from build123d import *

# Parameters (mm, degrees)
SKETCH1_W           = 40
SKETCH1_H           = 60
BOSS_EXTRUDE1_DEPTH = 3.05
SKETCH4_W           = 3.3
SKETCH4_H           = 52
SKETCH4_W_2         = 3
SKETCH4_H_2         = 0.8
CUT_EXTRUDE1_DEPTH  = 10
SKETCH7_R           = 8
CUT_EXTRUDE4_DEPTH  = 10
SKETCH8_R           = 1.5
CUT_EXTRUDE5_DEPTH  = 10
FILLET1_R           = 0.5


with BuildPart() as part:
    # Sketch1 → Boss-Extrude1 (new body)
    with BuildSketch(Plane(origin=(0, 0, 0), x_dir=(1, 0, 0), z_dir=(0, 1, 0))):
        with Locations((20, 30)):
            Rectangle(SKETCH1_W, SKETCH1_H)
    extrude(amount=BOSS_EXTRUDE1_DEPTH)

    # Sketch4 → Cut-Extrude1 (cut)
    with BuildSketch(Plane(origin=(0, 3.05, 0), x_dir=(1, 0, 0), z_dir=(0, 1, 0))):
        with Locations((20, 30)):
            Rectangle(SKETCH4_W, SKETCH4_H)
        with Locations((20, 57.6)):
            Rectangle(SKETCH4_W_2, SKETCH4_H_2)
    extrude(amount=-CUT_EXTRUDE1_DEPTH, mode=Mode.SUBTRACT)

    # Sketch7 → Cut-Extrude4 (cut)
    with BuildSketch(Plane(origin=(0, 3.05, 0), x_dir=(1, 0, 0), z_dir=(0, 1, 0))):
        with Locations((8, 35)):
            Circle(SKETCH7_R)
        with Locations((8, 49)):
            Circle(SKETCH7_R)
        with BuildLine():
            Line((8, 57), (0, 57))
            Line((0, 57), (0, 49))
            ThreePointArc((0, 49), (2.343145751, 54.656854249), (8, 57))
        make_face()
        with BuildLine():
            Line((16, 35), (16, 49))
            ThreePointArc((16, 49), (14.891439137, 44.936987987), (11.872983346, 42))
            ThreePointArc((11.872983346, 42), (14.891439137, 39.063012013), (16, 35))
        make_face()
        with BuildLine():
            ThreePointArc((4.127016654, 42), (1.108560863, 44.936987987), (0, 49))
            Line((0, 49), (0, 35))
            ThreePointArc((0, 35), (1.108560863, 39.063012013), (4.127016654, 42))
        make_face()
        with BuildLine():
            ThreePointArc((8, 27), (2.343145751, 29.343145751), (0, 35))
            Line((0, 35), (0, 27))
            Line((0, 27), (8, 27))
        make_face()
        with BuildLine():
            ThreePointArc((28.127016654, 42), (25.108560863, 44.936987987), (24, 49))
            Line((24, 49), (24, 35))
            ThreePointArc((24, 35), (25.108560863, 39.063012013), (28.127016654, 42))
        make_face()
        with Locations((32, 35)):
            Circle(SKETCH7_R)
        with Locations((32, 49)):
            Circle(SKETCH7_R)
        with BuildLine():
            Line((40, 35), (40, 49))
            ThreePointArc((40, 49), (38.891439137, 44.936987987), (35.872983346, 42))
            ThreePointArc((35.872983346, 42), (38.891439137, 39.063012013), (40, 35))
        make_face()
        with BuildLine():
            Line((40, 27), (40, 35))
            ThreePointArc((40, 35), (37.656854263, 29.343145764), (32.000000039, 27))
            Line((32.000000039, 27), (40, 27))
        make_face()
        with BuildLine():
            Line((40, 49), (40, 57))
            Line((40, 57), (32, 57))
            ThreePointArc((32, 57), (37.656854249, 54.656854249), (40, 49))
        make_face()
    extrude(amount=-CUT_EXTRUDE4_DEPTH, mode=Mode.SUBTRACT)

    # Sketch8 → Cut-Extrude5 (cut)
    with BuildSketch(Plane(origin=(0, 3.05, 0), x_dir=(1, 0, 0), z_dir=(0, 1, 0))):
        with BuildLine():
            ThreePointArc((9.5, 2.5), (6.939339828, 3.560660172), (8, 1))
            Line((8, 1), (8, 2.5))
            Line((8, 2.5), (9.5, 2.5))
        make_face()
        with BuildLine():
            Line((8, 2.5), (8, 1))
            ThreePointArc((8, 1), (9.060660172, 1.439339828), (9.5, 2.5))
            Line((9.5, 2.5), (8, 2.5))
        make_face()
        with Locations(Location((32, 2.5, 0), (0, 0, 270))):
            Circle(SKETCH8_R)
    extrude(amount=-CUT_EXTRUDE5_DEPTH, mode=Mode.SUBTRACT)

    # Fillet1
    fillet1_edges = [part.edges().sort_by_distance(p)[0] for p in [
        (0, 1.525, -27),
        (0, 1.525, -57),
        (40, 1.525, -57),
        (40, 1.525, -27),
        (0, 1.525, -60),
        (40, 1.525, -60),
    ]]
    fillet(fillet1_edges, radius=FILLET1_R)


solid = part.part
Verification items for the finished model (mm, model axes). A direction names the side the tool comes from. Give positions to 0.01 mm unless a question says otherwise; leave off trailing zeros. Write each loop counter-clockwise with the first axis right and the second up, starting at its lowest first coordinate (ties: lowest second). Pieces come first, ordered by that corner, then holes. Notation, with made-up numbers: M -28,-13 L -13,-13 A14 cw -13,8 Z; hole C 22,43.25 d7. An arc over 180 degrees is marked long. Put each result on its own line as item: value. Start each with the question number.
1. Scan lines: line 1 along Z through (x, y) = (20, 2); line 2 along X through (y, z) = (0.6, -2.5); line 3 along Z through (x, y) = (8, 1.4). Record each from-to range of solid material in increasing order. Write a range as [from, to].
2. Section check B-B (y = 2.25). Give the number of separate pieces and of enclosed holes in the cut face, and give its area (3 significant figures).
3. Section check C-C (z = -12.5). Record the cut outline in (x, y).
4. Draft check along Z on faces 1 (the face through (4, 2, -27)), 2 (the face through (20, 2, -60)), 3 (the face through (0, 2, -58)). Enter one of: +Z half, -Z half, draft (parallel to the pull), parting line (faces both ways), or undercut.
5. Go/stop test with flat-tipped pins: pin 1 Ø0.9 at (y, z) = (1.5, -45) entering from -X; pin 2 Ø1.5 at (y, z) = (2, -31) entering from +X; pin 3 Ø1.5 at (y, z) = (2.5, -39.5) entering from +X. Record where each tip stops, or that it passes through.
6. Set-up check for faces 4 (the face through (36, 2, -27)), 5 (the face through (0, 2, -13)), 6 (the face through (16, 2, -42)), 7 (the face through (20, 2, -58)): record each of +Z, -Z, +X, -X, +Y, -Y from which the full face is reachable in a straight line by a thin tool's end or side.
7. Section check A-A (z = -41). Record the cut outline in (x, y).
Answer list:
1. line 1: [-60, -58], [-57.2, -56], [-4, 0]
1. line 2: [0, 6.5], [9.5, 30.5], [33.5, 40]
1. line 3: [-60, -57], [-27, -4], [-1, 0]
2. separate pieces: 1
2. enclosed holes: 4
2. area: 1,310 mm2
3. outline: M 0,0 L 18.35,0 L 18.35,3.05 L 0,3.05 Z; M 21.65,0 L 40,0 L 40,3.05 L 21.65,3.05 Z
4. face 1: undercut
4. face 2: -Z half
4. face 3: draft
5. pin 1: x = 16
5. pin 2: x = 25.56
5. pin 3: x = 24
6. face 4: +X, +Y, -Y
6. face 5: +Z, -Z, -X, +Y, -Y
6. face 6: -X, +Y, -Y
6. face 7: +Y, -Y
7. outline: M 16,0 L 18.35,0 L 18.35,3.05 L 16,3.05 Z; M 21.65,0 L 24,0 L 24,3.05 L 21.65,3.05 Z
